For this review, take the finished solid that the model builds, in its own axes (mm). A direction names the side the tool comes from. Give positions to 0.01 mm unless a question says otherwise; leave off trailing zeros. Order: outer loops, then holes, each group sorted by start corner. A loop starts at its lowest first (then second) coordinate and runs counter-clockwise, first axis right, second up.
from build123d import *

# Parameters (mm, degrees)
SKETCH1_R           = 1.1303
SKETCH1_W           = 2.983921929
SKETCH1_H           = 4.98
BOSS_EXTRUDE1_DEPTH = 1
FILLET1_R           = 1


with BuildPart() as part:
    # Sketch1 → Boss-Extrude1 (new body)
    with BuildSketch(Plane.XY):
        Polygon((-26.65, 16.1), (-40.032188793, 16.1), (-40.032188793, -16.08), (-26.65, -16.08), (-26.65, -9.752186355), (4.81, -9.752186355), (4.81, -16.08), (40.590666929, -16.08), (40.590666929, -10.095824831), (30.822198497, -10.095824831), (30.822198497, 10.115824831), (40.590666929, 10.115824831), (40.590666929, 16.1), (4.81, 16.1), (4.81, 9.693936617), (-26.65, 9.693936617), align=None)
        with Locations((-37.532188793, 13.6)):
            Circle(SKETCH1_R, mode=Mode.SUBTRACT)
        with Locations((-37.532188793, -13.58)):
            Circle(SKETCH1_R, mode=Mode.SUBTRACT)
        with Locations((38.090666929, 13.6)):
            Circle(SKETCH1_R, mode=Mode.SUBTRACT)
        with Locations((38.090666929, -13.58)):
            Circle(SKETCH1_R, mode=Mode.SUBTRACT)
        with Locations((-3.751960965, 0)):
            Rectangle(SKETCH1_W, SKETCH1_H, mode=Mode.SUBTRACT)
        with BuildLine():
            Line((-32.190591627, 13.451742973), (-31.061789136, 13.451742973))
            ThreePointArc((-31.061789136, 13.451742973), (-29.086350608, 11.476304445), (-31.061789136, 9.500865917))
            Line((-31.061789136, 9.500865917), (-32.190591627, 9.500865917))
            ThreePointArc((-32.190591627, 9.500865917), (-34.166030155, 11.476304445), (-32.190591627, 13.451742973))
        make_face(mode=Mode.SUBTRACT)
    extrude(amount=BOSS_EXTRUDE1_DEPTH)

    # Fillet1
    fillet1_edges = [part.edges().sort_by_distance(p)[0] for p in [
        (40.590666929, 13.107912416, 1),
        (22.700333464, 16.1, 1),
        (40.590666929, -13.087912416, 1),
        (22.700333464, -16.08, 1),
        (-33.341094396, -16.08, 1),
        (-40.032188793, 0.01, 1),
        (-33.341094396, 16.1, 1),
    ]]
    fillet(fillet1_edges, radius=FILLET1_R - 0.0001)  # a hair under: the kernel refuses the full size


solid = part.part
1) Tool access review of faces 1 (the face through (0, 0, 1)), 2 (the face through (-29.087, 11.52, 0.493)): name each direction out of +Z, -Z, +X, -X, +Y, -Y from which nothing blocks a thin tool from reaching the whole face with its end or side.
Answer sheet:
face 1: +Z, +X, -X, +Y, -Y
face 2: +Z, -Z
2) We need section C-C on z = 0.8. Give the boundary of the cut face in (x, y).
Answer sheet:
outline: (-39.63, -15.68) - (-26.65, -15.68) - (-26.65, -9.75) - (4.81, -9.75) - (4.81, -15.68) - (40.19, -15.68) - (40.19, -10.1) - (30.82, -10.1) - (30.82, 10.12) - (40.19, 10.12) - (40.19, 15.7) - (4.81, 15.7) - (4.81, 9.69) - (-26.65, 9.69) - (-26.65, 15.7) - (-39.63, 15.7) - close; hole circle Ø2.26 at (-37.53, -13.58); hole circle Ø2.26 at (-37.53, 13.6); hole (-32.19, 9.5) - (-31.06, 9.5) arc R1.98 ccw to (-31.06, 13.45) - (-32.19, 13.45) arc R1.98 ccw to start; hole (-5.24, -2.49) - (-2.26, -2.49) - (-2.26, 2.49) - (-5.24, 2.49) - close; hole circle Ø2.26 at (38.09, -13.58); hole circle Ø2.26 at (38.09, 13.6)
3) Clearance check with flat-ended pins moving along their axes: pin 1 (0.5 mm diameter, centred on x = -13, z = 0.5, fed in from +Y); pin 2 (0.5 mm diameter, centred on x = 37, z = 0.5, fed in from +Y). State where each tip first meets the part, or that it passes through.
Answer sheet:
pin 1: stops at y = 9.69
pin 2: stops at y = 16.07
4) To check wall thickness, follow line 1 (Y direction, x = -5, z = 0.9); line 2 (Y direction, x = -17.5, z = 0.1); line 3 (X direction, y = -0.5, z = 0.9). State the ranges of each line that lie inside material, in increasing order.
Answer sheet:
line 1: y = -9.75 to -2.49, 2.49 to 9.69
line 2: y = -9.75 to 9.69
line 3: x = -39.47 to -5.24, -2.26 to 30.82
5) We need section A-A on y = -13.58. Count the separate pieces of the cut face and the enclosed holes in it, then the cut area to 3 significant figures.
Answer sheet:
separate pieces: 4
enclosed holes: 0
area: 44.2 mm2
6) Draft analysis for pull direction X (two halves, no side actions). For faces 3 (the face through (37.258, 14.364, 0.493)), 4 (the face through (0, 0, 0)), 5 (the face through (-37.68, 14.72, 0.49)), state which applies: +X half, -X half, draft (parallel to the pull), parting line (faces both ways), or undercut.
Answer sheet:
face 3: undercut
face 4: draft
face 5: undercut
